from build123d import *

# Parameters (mm, degrees)
SKETCH1_R                       = 0.75
BASE_FLANGE1_DEPTH              = 0.43
EDGE_FLANGE1_STRIP_CUT_DEPTH    = 1
EDGE_FLANGE1_DEPTH              = 1
FILLET1_RADIUS                  = 0.5
FILLET1_LENGTH                  = 0.43
CIRPATTERN1_COUNT               = 8
FILLET1_OF_CIRPATTERN1_2_RADIUS = 0.5
FILLET1_OF_CIRPATTERN1_2_LENGTH = 0.43
FILLET1_OF_CIRPATTERN1_3_RADIUS = 0.5
FILLET1_OF_CIRPATTERN1_3_LENGTH = 0.43
FILLET1_OF_CIRPATTERN1_4_RADIUS = 0.5
FILLET1_OF_CIRPATTERN1_4_LENGTH = 0.43
FILLET1_OF_CIRPATTERN1_5_RADIUS = 0.5
FILLET1_OF_CIRPATTERN1_5_LENGTH = 0.43
FILLET1_OF_CIRPATTERN1_6_RADIUS = 0.5
FILLET1_OF_CIRPATTERN1_6_LENGTH = 0.43
EDGE_FLANGE2_STRIP_W            = 3.1932
EDGE_FLANGE2_STRIP_H            = 0.43
EDGE_FLANGE2_STRIP_CUT_DEPTH    = 1.25
EDGE_FLANGE2_RELIEF_W           = 3.4082
EDGE_FLANGE2_RELIEF_H           = 0.215
EDGE_FLANGE2_RELIEF_CUT_DEPTH   = 0.43
EDGE_FLANGE2_DEPTH              = 1.25
TAB1_DEPTH                      = 0.43
FILLET2_R                       = 0.25


# Sheet-metal steps are written as plain solids
with BuildPart() as part:
    # Sketch1 → Base-Flange1 (new body)
    with BuildSketch(Plane(origin=(0, 0, 0), x_dir=(1, 0, 0), z_dir=(0, 1, 0))):
        with BuildLine():
            Line((5.75, 0.5), (2.414213562, 0.5))
            ThreePointArc((2.414213562, 0.5), (1.952273796, 0.808658284), (2.060660172, 1.353553391))
            Line((2.060660172, 1.353553391), (4.419417382, 3.712310601))
            Line((4.419417382, 3.712310601), (3.712310601, 4.419417382))
            Line((3.712310601, 4.419417382), (1.353553391, 2.060660172))
            Line((1.353553391, 2.060660172), (-1.353553391, 2.060660172))
            Line((-1.353553391, 2.060660172), (-3.712310601, 4.419417382))
            Line((-3.712310601, 4.419417382), (-4.419417382, 3.712310601))
            Line((-4.419417382, 3.712310601), (-2.060660172, 1.353553391))
            ThreePointArc((-2.060660172, 1.353553391), (-1.952273796, 0.808658284), (-2.414213562, 0.5))
            Line((-2.414213562, 0.5), (-5.75, 0.5))
            Line((-5.75, 0.5), (-5.75, -0.5))
            Line((-5.75, -0.5), (-2.414213562, -0.5))
            ThreePointArc((-2.414213562, -0.5), (-1.952273796, -0.808658284), (-2.060660172, -1.353553391))
            Line((-2.060660172, -1.353553391), (-4.419417382, -3.712310601))
            Line((-4.419417382, -3.712310601), (-3.712310601, -4.419417382))
            Line((-3.712310601, -4.419417382), (-1.353553391, -2.060660172))
            Line((-1.353553391, -2.060660172), (1.353553391, -2.060660172))
            Line((1.353553391, -2.060660172), (3.712310601, -4.419417382))
            Line((3.712310601, -4.419417382), (4.419417382, -3.712310601))
            Line((4.419417382, -3.712310601), (2.060660172, -1.353553391))
            ThreePointArc((2.060660172, -1.353553391), (1.952273796, -0.808658284), (2.414213562, -0.5))
            Line((2.414213562, -0.5), (5.75, -0.5))
            Line((5.75, -0.5), (5.75, 0.5))
        make_face()
        with Locations(Location((0, 0, 0), (0, 0, 270))):
            Circle(SKETCH1_R, mode=Mode.SUBTRACT)
    extrude(amount=-BASE_FLANGE1_DEPTH)

    # Edge-Flange1 strip (across the edge) → Edge-Flange1 strip cut (cut)
    with BuildSketch(Plane(origin=(4.419417382, 0, -3.712310601), x_dir=(-0.7053843046066381, 0.0697564737441289, 0.7053843046066409), z_dir=(-0.707106781186549, 0, -0.7071067811865462))):
        Polygon((-2.530199428, -0.254121237), (0.655222098, -0.476867609), (0.685217381, -0.047915067), (-2.500204144, 0.174831305), align=None)
    edge_flange1_strip_cut = extrude(amount=EDGE_FLANGE1_STRIP_CUT_DEPTH, mode=Mode.SUBTRACT)

    # Edge-Flange1 section (across the edge) → Edge-Flange1 (add)
    with BuildSketch(Plane(origin=(4.419417382, 0, -3.712310601), x_dir=(-0.7053843046066381, 0.0697564737441289, 0.7053843046066409), z_dir=(-0.707106781186549, 0, -0.7071067811865462))):
        with BuildLine():
            Line((-0.43, 0.686890612), (-0.43, 4.599018513))
            Line((-0.43, 4.599018513), (0, 4.599018513))
            Line((0, 4.599018513), (0, 0.686890612))
            ThreePointArc((0, 0.686890612), (0.197884863, 0.18453062), (0.685217381, -0.047915067))
            Line((0.685217381, -0.047915067), (0.655222098, -0.476867609))
            ThreePointArc((0.655222098, -0.476867609), (-0.116597228, -0.108728674), (-0.43, 0.686890612))
        make_face()
    edge_flange1 = extrude(amount=EDGE_FLANGE1_DEPTH)

    # Fillet1: full round fillet: the end face becomes a half cylinder, R = half its width
    fillet1_face = Plane((4.444369473, 4.572817893, -4.444369473), x_dir=(0.705384304607, -0.069756473744, -0.705384304607), z_dir=(0.049325275616, 0.99756405026, -0.049325275616))  # on the end face: x along it, z out of the body
    fillet1_slab = fillet1_face.offset(-FILLET1_RADIUS / 2) * Box(FILLET1_LENGTH, 2 * FILLET1_RADIUS, FILLET1_RADIUS, mode=Mode.PRIVATE)  # the body's end, R deep
    fillet1_round = Plane((4.419706835, 4.074035868, -4.419706835), x_dir=(0.049325275616, 0.99756405026, -0.049325275616), z_dir=(0.705384304607, -0.069756473744, -0.705384304607)) * Cylinder(FILLET1_RADIUS, FILLET1_LENGTH, mode=Mode.PRIVATE)  # its axis R under the face
    add(fillet1_slab - fillet1_round, mode=Mode.SUBTRACT)

    # CirPattern1: Edge-Flange1 strip cut, Edge-Flange1 ×8 about axis, 2 skipped
    cirpattern1_axis = Axis((0, -0.43, 0), (0, 1, 0))
    add([edge_flange1_strip_cut.rotate(cirpattern1_axis, i * 360 / CIRPATTERN1_COUNT) for i in range(1, CIRPATTERN1_COUNT) if i not in (1, 5)], mode=Mode.SUBTRACT)
    add([edge_flange1.rotate(cirpattern1_axis, i * 360 / CIRPATTERN1_COUNT) for i in range(1, CIRPATTERN1_COUNT) if i not in (1, 5)])

    # Fillet1 of CirPattern1 2: full round fillet: the end face becomes a half cylinder, R = half its width
    fillet1_of_cirpattern1_2_face = Plane((-4.444369473, 4.572817893, -4.444369473), x_dir=(-0.705384304607, -0.069756473744, -0.705384304607), z_dir=(-0.049325275616, 0.99756405026, -0.049325275616))  # on the end face: x along it, z out of the body
    fillet1_of_cirpattern1_2_slab = fillet1_of_cirpattern1_2_face.offset(-FILLET1_OF_CIRPATTERN1_2_RADIUS / 2) * Box(FILLET1_OF_CIRPATTERN1_2_LENGTH, 2 * FILLET1_OF_CIRPATTERN1_2_RADIUS, FILLET1_OF_CIRPATTERN1_2_RADIUS, mode=Mode.PRIVATE)  # the body's end, R deep
    fillet1_of_cirpattern1_2_round = Plane((-4.419706835, 4.074035868, -4.419706835), x_dir=(-0.049325275616, 0.99756405026, -0.049325275616), z_dir=(-0.705384304607, -0.069756473744, -0.705384304607)) * Cylinder(FILLET1_OF_CIRPATTERN1_2_RADIUS, FILLET1_OF_CIRPATTERN1_2_LENGTH, mode=Mode.PRIVATE)  # its axis R under the face
    add(fillet1_of_cirpattern1_2_slab - fillet1_of_cirpattern1_2_round, mode=Mode.SUBTRACT)

    # Fillet1 of CirPattern1 3: full round fillet: the end face becomes a half cylinder, R = half its width
    fillet1_of_cirpattern1_3_face = Plane((-6.285287585, 4.572817893, 0), x_dir=(-0.99756405026, -0.069756473744, 0), z_dir=(-0.069756473744, 0.99756405026, 0))  # on the end face: x along it, z out of the body
    fillet1_of_cirpattern1_3_slab = fillet1_of_cirpattern1_3_face.offset(-FILLET1_OF_CIRPATTERN1_3_RADIUS / 2) * Box(FILLET1_OF_CIRPATTERN1_3_LENGTH, 2 * FILLET1_OF_CIRPATTERN1_3_RADIUS, FILLET1_OF_CIRPATTERN1_3_RADIUS, mode=Mode.PRIVATE)  # the body's end, R deep
    fillet1_of_cirpattern1_3_round = Plane((-6.250409348, 4.074035868, 0), x_dir=(-0.069756473744, 0.99756405026, 0), z_dir=(-0.99756405026, -0.069756473744, 0)) * Cylinder(FILLET1_OF_CIRPATTERN1_3_RADIUS, FILLET1_OF_CIRPATTERN1_3_LENGTH, mode=Mode.PRIVATE)  # its axis R under the face
    add(fillet1_of_cirpattern1_3_slab - fillet1_of_cirpattern1_3_round, mode=Mode.SUBTRACT)

    # Fillet1 of CirPattern1 4: full round fillet: the end face becomes a half cylinder, R = half its width
    fillet1_of_cirpattern1_4_face = Plane((-4.444369473, 4.572817893, 4.444369473), x_dir=(-0.705384304607, -0.069756473744, 0.705384304607), z_dir=(-0.049325275616, 0.99756405026, 0.049325275616))  # on the end face: x along it, z out of the body
    fillet1_of_cirpattern1_4_slab = fillet1_of_cirpattern1_4_face.offset(-FILLET1_OF_CIRPATTERN1_4_RADIUS / 2) * Box(FILLET1_OF_CIRPATTERN1_4_LENGTH, 2 * FILLET1_OF_CIRPATTERN1_4_RADIUS, FILLET1_OF_CIRPATTERN1_4_RADIUS, mode=Mode.PRIVATE)  # the body's end, R deep
    fillet1_of_cirpattern1_4_round = Plane((-4.419706835, 4.074035868, 4.419706835), x_dir=(-0.049325275616, 0.99756405026, 0.049325275616), z_dir=(-0.705384304607, -0.069756473744, 0.705384304607)) * Cylinder(FILLET1_OF_CIRPATTERN1_4_RADIUS, FILLET1_OF_CIRPATTERN1_4_LENGTH, mode=Mode.PRIVATE)  # its axis R under the face
    add(fillet1_of_cirpattern1_4_slab - fillet1_of_cirpattern1_4_round, mode=Mode.SUBTRACT)

    # Fillet1 of CirPattern1 5: full round fillet: the end face becomes a half cylinder, R = half its width
    fillet1_of_cirpattern1_5_face = Plane((4.444369473, 4.572817893, 4.444369473), x_dir=(0.705384304607, -0.069756473744, 0.705384304607), z_dir=(0.049325275616, 0.99756405026, 0.049325275616))  # on the end face: x along it, z out of the body
    fillet1_of_cirpattern1_5_slab = fillet1_of_cirpattern1_5_face.offset(-FILLET1_OF_CIRPATTERN1_5_RADIUS / 2) * Box(FILLET1_OF_CIRPATTERN1_5_LENGTH, 2 * FILLET1_OF_CIRPATTERN1_5_RADIUS, FILLET1_OF_CIRPATTERN1_5_RADIUS, mode=Mode.PRIVATE)  # the body's end, R deep
    fillet1_of_cirpattern1_5_round = Plane((4.419706835, 4.074035868, 4.419706835), x_dir=(0.049325275616, 0.99756405026, 0.049325275616), z_dir=(0.705384304607, -0.069756473744, 0.705384304607)) * Cylinder(FILLET1_OF_CIRPATTERN1_5_RADIUS, FILLET1_OF_CIRPATTERN1_5_LENGTH, mode=Mode.PRIVATE)  # its axis R under the face
    add(fillet1_of_cirpattern1_5_slab - fillet1_of_cirpattern1_5_round, mode=Mode.SUBTRACT)

    # Fillet1 of CirPattern1 6: full round fillet: the end face becomes a half cylinder, R = half its width
    fillet1_of_cirpattern1_6_face = Plane((6.285287585, 4.572817893, 0), x_dir=(0.99756405026, -0.069756473744, 0), z_dir=(0.069756473744, 0.99756405026, 0))  # on the end face: x along it, z out of the body
    fillet1_of_cirpattern1_6_slab = fillet1_of_cirpattern1_6_face.offset(-FILLET1_OF_CIRPATTERN1_6_RADIUS / 2) * Box(FILLET1_OF_CIRPATTERN1_6_LENGTH, 2 * FILLET1_OF_CIRPATTERN1_6_RADIUS, FILLET1_OF_CIRPATTERN1_6_RADIUS, mode=Mode.PRIVATE)  # the body's end, R deep
    fillet1_of_cirpattern1_6_round = Plane((6.250409348, 4.074035868, 0), x_dir=(0.069756473744, 0.99756405026, 0), z_dir=(0.99756405026, -0.069756473744, 0)) * Cylinder(FILLET1_OF_CIRPATTERN1_6_RADIUS, FILLET1_OF_CIRPATTERN1_6_LENGTH, mode=Mode.PRIVATE)  # its axis R under the face
    add(fillet1_of_cirpattern1_6_slab - fillet1_of_cirpattern1_6_round, mode=Mode.SUBTRACT)

    # Edge-Flange2 strip (across the edge) → Edge-Flange2 strip cut (cut)
    with BuildSketch(Plane(origin=(0.625, 0, -2.060660172), x_dir=(0, 0, 1), z_dir=(-1, 0, 0))):
        with Locations((-0.86, -0.215)):
            Rectangle(EDGE_FLANGE2_STRIP_W, EDGE_FLANGE2_STRIP_H)
    edge_flange2_strip_cut = extrude(amount=EDGE_FLANGE2_STRIP_CUT_DEPTH, mode=Mode.SUBTRACT)

    # Edge-Flange2 relief (on the sheet) → Edge-Flange2 relief cut (cut)
    with BuildSketch(Plane(origin=(0.625, 0, -1.324060172), x_dir=(0, 0, 1), z_dir=(0, 1, 0))):
        with Locations((-1.4891, 0.1075)):
            Rectangle(EDGE_FLANGE2_RELIEF_W, EDGE_FLANGE2_RELIEF_H)
        with Locations((-1.4891, -1.3575)):
            Rectangle(EDGE_FLANGE2_RELIEF_W, EDGE_FLANGE2_RELIEF_H)
    edge_flange2_relief_cut = extrude(amount=-EDGE_FLANGE2_RELIEF_CUT_DEPTH, mode=Mode.SUBTRACT)

    # Edge-Flange2 section (across the edge) → Edge-Flange2 (add)
    with BuildSketch(Plane(origin=(0.625, 0, -2.060660172), x_dir=(0, 0, 1), z_dir=(-1, 0, 0))):
        with BuildLine():
            Line((-0.43, 0.7366), (-0.43, 4.5))
            Line((-0.43, 4.5), (0, 4.5))
            Line((0, 4.5), (0, 0.7366))
            ThreePointArc((0, 0.7366), (0.215745145, 0.215745145), (0.7366, 0))
            Line((0.7366, 0), (0.7366, -0.43))
            ThreePointArc((0.7366, -0.43), (-0.088310771, -0.088310771), (-0.43, 0.7366))
        make_face()
    edge_flange2 = extrude(amount=EDGE_FLANGE2_DEPTH)

    # Sketch13 → Tab1 (add)
    with BuildSketch(Plane.XY.offset(-2.060660172)):
        with BuildLine():
            ThreePointArc((-1.411764706, 6.202941176), (0, 3.85), (1.411764706, 6.202941176))
            ThreePointArc((1.411764706, 6.202941176), (0.972058824, 6.336764706), (0.838235294, 5.897058824))
            ThreePointArc((0.838235294, 5.897058824), (0, 4.5), (-0.838235294, 5.897058824))
            ThreePointArc((-0.838235294, 5.897058824), (-0.972058824, 6.336764706), (-1.411764706, 6.202941176))
        make_face()
    tab1 = extrude(amount=-TAB1_DEPTH)

    # Mirror1: Edge-Flange2 strip cut, Edge-Flange2 relief cut, Edge-Flange2, Tab1 across plane
    add(edge_flange2_strip_cut.mirror(Plane.XY), mode=Mode.SUBTRACT)
    add(edge_flange2_relief_cut.mirror(Plane.XY), mode=Mode.SUBTRACT)
    add(edge_flange2.mirror(Plane.XY))
    add(tab1.mirror(Plane.XY))

    # Fillet2
    fillet2_edges = [part.edges().sort_by_distance(p)[0] for p in [
        (1.353553391, -0.215, 2.060660172),
        (-1.353553391, -0.215, 2.060660172),
        (-1.353553391, -0.215, -2.060660172),
        (1.353553391, -0.215, -2.060660172),
    ]]
    fillet(fillet2_edges, radius=FILLET2_R)


solid = part.part
Check sheet for the modelled part. Datum: model origin and axes. Units: mm. A direction names the side the tool comes from. Give positions to 0.01 mm unless a question says otherwise; leave off trailing zeros. Loops run counter-clockwise (first coordinate to the right, second up) from the corner with the lowest first, then second, coordinate; pieces in that order, holes last. Notation, with made-up numbers: M 18,-12.5 L 65,-12.5 A18 cw 65,-6.5 Z; hole C 10,7 d9. An arc over 180 degrees is marked long. Answer as a JSON object with one key per item and string values. Group by question number.
Q1. Cross-section at A-A on y = 5.45. Record the cut outline in (x, z).
Q2. Access from +Z, -Z, +X, -X, +Y, -Y to the whole of each face (thin tool, end or side, straight path). Record for faces 1 (the flat face through (-4.2, 2.7, 4.2)), 2 (the flat face through (-0.625, 1.8, -2.3)), 3 (the flat face through (6, 1, -0.5)), 4 (the flat face through (-6, 1, 0.5)), 5 (the flat face through (-5.936, 2.664, -0.007)).
Q3. Material ranges on line 1 along X through (y, z) = (5.45, 2.4); line 2 along Y through (x, z) = (1.75, -0.5); line 3 along X through (y, z) = (-0.2, 0), recorded low to high. Write a range as [from, to].
Q4. Cross-section at C-C on x = 3. Record the cut outline in (y, z), then the cut area to 3 significant figures.
Q5. Release check for a two-part mould opening along X. For faces 6 (the cylindrical face through (-4.141, -0.125, 4.131)), 7 (the flat face through (4.5, 2.6, -4.5)), 8 (the flat face through (-6, 1, -0.5)), 9 (the flat face through (0.625, 1.8, -2.3)) record: released by +X, released by -X, zero draft, split by the parting line, or undercut.
Q6. Cross-section at D-D on y = 1.5. Give the number of separate pieces and of enclosed holes in the cut face, then the cut area to 3 significant figures.
Q7. Go/stop test with flat-tipped pins: P1, Ø3, axis at y = 1.5, z = -0.5, coming from the -X side; P2, Ø3.5, axis at x = 0, y = 5, coming from the +Z side; P3, Ø3.5, axis at x = 0.5, y = 2.5, coming from the -Z side. Record where each tip stops, or that it passes through.
Q8. Cross-section at B-B on z = 0. Record the cut outline in (x, y).
Evaluation:
{
 "1": {"outline": "M -1.6,-2.49 L -0.95,-2.49 L -0.95,-2.06 L -1.6,-2.06 Z; M -1.6,2.06 L -0.95,2.06 L -0.95,2.49 L -1.6,2.49 Z; M 0.95,-2.49 L 1.6,-2.49 L 1.6,-2.06 L 0.95,-2.06 Z; M 0.95,2.06 L 1.6,2.06 L 1.6,2.49 L 0.95,2.49 Z"},
 "2": {"face 1": "+Y", "face 2": "-Z, -Y", "face 3": "+X, +Y, -Y", "face 4": "-X, +Y, -Y", "face 5": "+Z, -Z, +Y"},
 "3": {"line 1": "x = [-1.6, -0.95], [0.95, 1.6]", "line 2": "y = [-0.43, 0]", "line 3": "x = [-5.76, -0.75], [0.75, 5.76]"},
 "4": {"outline": "M -0.43,-3.71 L 0,-3.71 L 0,-2.29 L -0.43,-2.29 Z; M -0.43,-0.5 L 0,-0.5 L 0,0.5 L -0.43,0.5 Z; M -0.43,2.29 L 0,2.29 L 0,3.71 L -0.43,3.71 Z", "area": "1.65 mm2"},
 "5": {"face 6": "released by -X", "face 7": "released by +X", "face 8": "zero draft", "face 9": "undercut"},
 "6": {"separate pieces": "8", "enclosed holes": "0", "area": "3.66 mm2"},
 "7": {"P1": "stops at x = -6.39", "P2": "stops at z = 2.49", "P3": "stops at z = -2.49"},
 "8": {"outline": "M -6.5,4.56 L -6.23,0.66 A1.17 ccw -5.06,-0.43 L -0.75,-0.43 L -0.75,0 L -5.06,0 A0.74 cw -5.8,0.69 L -6.07,4.59 Z; M 0.75,-0.43 L 5.06,-0.43 A1.17 ccw 6.23,0.66 L 6.5,4.56 L 6.07,4.59 L 5.8,0.69 A0.74 cw 5.06,0 L 0.75,0 Z"}
}
